Design review of the part shown in the three views and the two pictorial views. Dimensions are in mm from the part's minimum x, y and z. A direction names the side the tool comes from. Coordinates: 2 decimals unless noted, no trailing zeros. Loops run counter-clockwise (first coordinate to the right, second up) from the corner with the lowest first, then second, coordinate; pieces in that order, holes last. Notation, with made-up numbers: M -6,22.25 L 10,22.25 A29 ccw 10,55.25 Z; hole C -20,-0.5 d4. An arc over 180 degrees is marked long. Use one line per item in the form item = value.
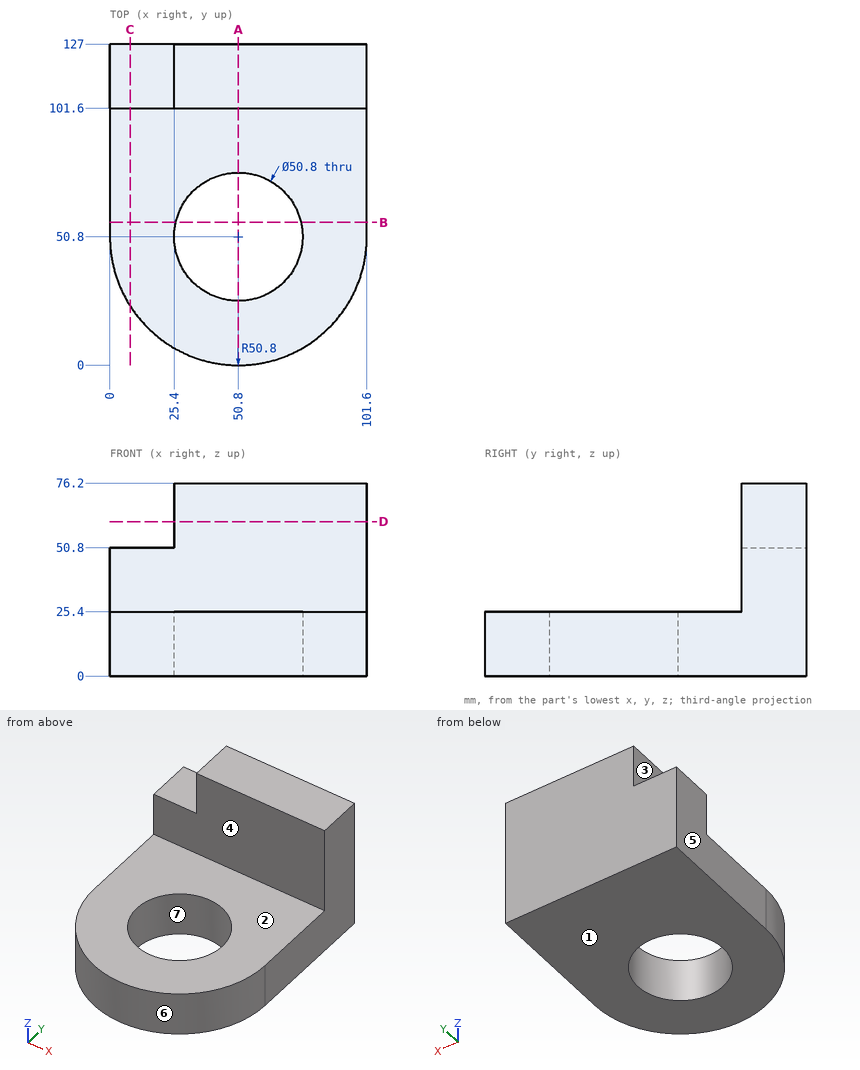
1. Add section A-A (x = 50.8). State the section outline as (y, z) points, then the cut area to 3 significant figures.
Response values:
outline = M 0,0 L 25.4,0 L 25.4,25.4 L 0,25.4 Z; M 76.2,0 L 127,0 L 127,76.2 L 101.6,76.2 L 101.6,25.4 L 76.2,25.4 Z
area = 3,230 mm^2
2. Add section D-D (z = 61). State the section outline as (x, y) points.
Response values:
outline = M 25.4,101.6 L 101.6,101.6 L 101.6,127 L 25.4,127 Z
3. Insertion check: P1, Ø10, axis at x = 38.5, z = 31, coming from the -Y side; P2, Ø7.5, axis at y = 118, z = 58.5, coming from the -X side; P3, Ø2, axis at x = 54.5, y = 17, coming from the +Z side. Each pin has a flat end and moves straight along its axis. Give the tip position at first contact, or say it passes through.
Response values:
P1 = 101.6
P2 = 25.4
P3 = 25.4
4. Wall thickness on line 1 along Y through (x, z) = (50.8, 8); line 2 along X through (y, z) = (50, 19); line 3 along Z through (x, y) = (91, 87.5): over which ranges is each line inside the solid? List them lowest first. Write a range as from..to.
Response values:
line_1 = 0..25.4, 76.2..127
line_2 = 0.01..25.41, 76.19..101.59
line_3 = 0..25.4
5. Machinability: for the marked faces 1, 2 and 3, which of the approach directions +Z, -Z, +X, -X, +Y, -Y give a long, thin tool a straight path to every point of the face, cutting with its end or side? Answer none if there is none.
Response values:
face_1 = -Z, +X, -X, +Y, -Y
face_2 = +Z, +X, -X, -Y
face_3 = +Z, -X, +Y, -Y
6. Add section B-B (y = 56.5). State the section outline as (x, z) points, then the cut area to 3 significant figures.
Response values:
outline = M 0,0 L 26.05,0 L 26.05,25.4 L 0,25.4 Z; M 75.55,0 L 101.6,0 L 101.6,25.4 L 75.55,25.4 Z
area = 1,320 mm^2
7. The part is to be moulded in two halves that separate along X. For the marked faces 4, 5, 6 and 7, say which applies: pulls with the +X half, pulls with the -X half, needs draft (parallel to the pull), parting line crosses it, or undercut.
Response values:
face_4 = needs draft
face_5 = pulls with the -X half
face_6 = parting line crosses it
face_7 = undercut
8. Add section C-C (x = 8). State the section outline as (y, z) points.
Response values:
outline = M 23.44,0 L 127,0 L 127,50.8 L 101.6,50.8 L 101.6,25.4 L 23.44,25.4 Z
